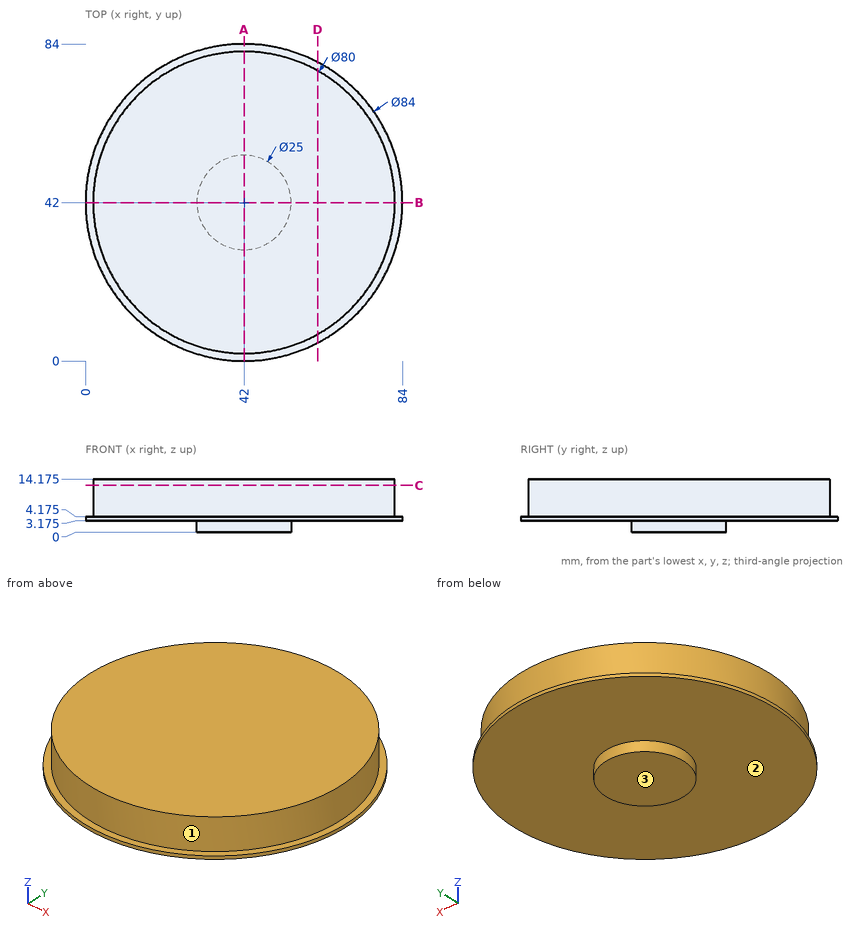
Here's the drawing with two shaded views (mm, measured from the low corner). I have some questions. A direction names the side the tool comes from. Give positions to 0.01 mm unless a question says otherwise; leave off trailing zeros. Loops run counter-clockwise (first coordinate to the right, second up) from the corner with the lowest first, then second, coordinate; pieces in that order, holes last. Notation, with made-up numbers: M -10.5,65.5 L 8.5,65.5 A21 cw 8.5,104.5 Z; hole C 73.5,37 d4. An arc over 180 degrees is marked long. One line per item, written item: value.
(1) Suppose I cut it at C-C on z = 12.5. List the corners of the cut face in (x, y) for me, plus the area to 3 significant figures.
Returned:
outline: C 42,42 d80
area: 5,030 mm^2
(2) I need wall thicknesses on line 1 (Z direction, x = 18, y = 45) (3 decimals); line 2 (Z direction, x = 27.5, y = 80) (3 decimals); line 3 (Y direction, x = 32.5, z = 3.5). Which ranges of each line are inside material? Lowest first, please.
Returned:
line 1: 3.175 to 14.175
line 2: 3.175 to 4.175
line 3: 1.09 to 82.91
(3) Which directions (+Z, -Z, +X, -X, +Y, -Y) give clear straight access to the entire face, cutting with the end or side of a thin tool? Please do the marked faces 1, 2 and 3.
Returned:
face 1: +Z
face 2: -Z
face 3: -Z, +X, -X, +Y, -Y
(4) Suppose I cut it at D-D on x = 61.5. List the corners of the cut face in (y, z) for me (3 decimals).
Returned:
outline: M 4.801,3.175 L 79.199,3.175 L 79.199,4.175 L 76.925,4.175 L 76.925,14.175 L 7.075,14.175 L 7.075,4.175 L 4.801,4.175 Z
(5) Will these pins go through, and if not, where does the flat tip stop? pin 1 (8 mm diameter, centred on x = 51, z = 9.5, fed in from +Y); pin 2 (8 mm diameter, centred on y = 48.5, z = 8, fed in from +X); pin 3 (1 mm diameter, centred on x = 45, y = 35.5, fed in from -Z); pin 4 (5 mm diameter, centred on y = 18, z = 10, fed in from +X).
Returned:
pin 1: y = 81.69
pin 2: x = 83.66
pin 3: z = 0
pin 4: x = 75.73
(6) Suppose I cut it at A-A on x = 42. List the corners of the cut face in (y, z) for me (3 decimals), plus the area to 3 significant figures.
Returned:
outline: M 0,3.175 L 29.5,3.175 L 29.5,0 L 54.5,0 L 54.5,3.175 L 84,3.175 L 84,4.175 L 82,4.175 L 82,14.175 L 2,14.175 L 2,4.175 L 0,4.175 Z
area: 963 mm^2
